For this review, take the finished solid that the model builds, in its own axes (mm). Face numbers are marked on the shaded views. A direction names the side the tool comes from. Round coordinates to 2 decimals unless told otherwise and drop trailing zeros. Loops run counter-clockwise (first coordinate to the right, second up) from the corner with the lowest first, then second, coordinate; pieces in that order, holes last. Notation, with made-up numbers: M -34,64 L 7,64 A11 ccw 7,70 Z; hole C -34,8.25 d11. An arc over 180 degrees is marked long. One line per question, with ' | ' between items. Start each with the question number.
1) We need section C-C (z = 24.5). Give the boundary of the cut face in (x, y).
2) We need section B-B (x = 10). Give the boundary of the cut face in (y, z), and give its area (3 significant figures).
3) For the marked faces 1, 2, 3 and 4, list the 3-axis set-ups (+Z, -Z, +X, -X, +Y, -Y) from which the entire face can be reached by the end or side of a thin tool; tool diameter is ignored.
4) For pin 1 Ø18.5 at (x, z) = (53.5, 31.5) entering from +Y; pin 2 Ø1.5 at (x, y) = (33.5, 7) entering from +Z; pin 3 Ø8.5 at (x, y) = (9.5, 6) entering from +Z, all flat-tipped, find the tip position at first contact; note any pin that passes through.
5) For probe 1 along Y at (x, z) = (10, 3); probe 2 along Z at (x, y) = (37, 75); probe 3 along Y at (x, z) = (17, 35), list the stretches that pass through material, from the lowest coordinate up. Write a range as from..to.
6) We need section D-D (z = 4). Give the boundary of the cut face in (x, y), and give its area (3 significant figures).
7) We need section A-A (y = 80). Give the boundary of the cut face in (x, z).
Autodesk Inventor part; units mm, degrees
ref_plane "YZ Plane" through (0, 0, 0) normal (1, 0, 0) x (0, 1, 0)
ref_plane "XZ Plane" through (0, 0, 0) normal (0, 1, 0) x (-1, 0, 0)
ref_plane "XY Plane" through (0, 0, 0) normal (0, 0, 1) x (1, 0, 0)
sketch "Sketch1" plane through (0, 0, 0) normal (0, 0, 1) x (1, 0, 0)
  line L0 (0, 0) -> (70, 0)
  line L1 (70, 0) -> (70, 90)
  line L2 (70, 90) -> (0, 90)
  line L3 (0, 90) -> (0, 0)
  dimension "d0" = 70
  dimension "d1" = 90
extrude "Extrusion1" add sketch "Sketch1" along normal blind 5
sketch "Sketch2" plane through (0, 0, 5) normal (0, 0, 1) x (1, 0, 0)
  circle A0 centre (35, 20) radius 12.5
  point P0 (0, 0)
  dimension "d4" = 25
extrude "Extrusion2" add sketch "Sketch2" along normal blind 40
sketch "Sketch3" plane through (35, 20, 45) normal (0, 0, 1) x (1, 0, 0)
  circle A0 centre (0, 0) radius 2.7
  point P0 (-35, -20)
  dimension "d7" = 5.4
extrude "Extrusion3" cut sketch "Sketch3" against normal blind 25
chamfer "Chamfer1" distance 4 angle 45 1 edges at (22.5, 20, 45) measured on face at (44.0861, 18.7875, 45)
sketch "Sketch4" plane through (0, 0, 5) normal (0, 0, 1) x (1, 0, 0)
  line L0 (0, 0) -> (70, 0)
  line L1 (32, 0) -> (38, 0)
  line L2 (38, 0) -> (38, 14)
  line L3 (38, 14) -> (32, 14)
  line L4 (32, 14) -> (32, 0)
  dimension "d13" = 6
  dimension "d14" = 14
extrude "Extrusion4" add sketch "Sketch4" along normal blind 36
chamfer "Chamfer2" distance 6 angle 45 1 edges at (35, 0, 41) measured on face at (35.3363, 2.5136, 41)
sketch "Sketch5" plane through (0, 0, 5) normal (0, 0, 1) x (1, 0, 0)
  line L0 (32, 72) -> (38, 72)
  line L1 (38, 72) -> (38, 27)
  line L2 (38, 27) -> (32, 27)
  line L3 (32, 27) -> (32, 72)
  line L4 (70, 0) -> (70, 90)
  line L5 (70, 23) -> (42, 23)
  line L6 (42, 23) -> (42, 17)
  line L7 (42, 17) -> (70, 17)
  line L8 (70, 17) -> (70, 23)
  line L9 (0, 90) -> (0, 0)
  line L10 (0, 23) -> (25.872, 23)
  line L11 (25.872, 23) -> (25.872, 17)
  line L12 (25.872, 17) -> (0, 17)
  line L13 (0, 17) -> (0, 23)
  dimension "d20" = 6
  dimension "d21" = 45
  dimension "d22" = 28
  dimension "d23" = 6
extrude "Extrusion5" add sketch "Sketch5" along normal blind 36
chamfer "Chamfer3" distance 20 angle 45 1 edges at (70, 20, 41) measured on face at (62.5, 20, 41)
chamfer "Chamfer4" distance 20 angle 45 1 edges at (0, 20, 41) measured on face at (7.5136, 20.3363, 41)
chamfer "Chamfer5" distance 35 angle 45 1 edges at (35, 72, 41) measured on face at (34, 72, 17)
sketch "Sketch6" plane through (0, 0, 5) normal (0, 0, 1) x (1, 0, 0)
  circle A0 centre (10, 7) radius 2.5
  circle A1 centre (60, 7) radius 2.5
  circle A2 centre (10, 80) radius 2.5
  circle A3 centre (60, 80) radius 2.5
  circle A4 centre (10, 45) radius 2.5
  circle A5 centre (60, 45) radius 2.5
  point P0 (0, 0)
  dimension "d35" = 5
  dimension "d36" = 5
  dimension "d37" = 5
  dimension "d38" = 5
  dimension "d39" = 5
  dimension "d40" = 5
extrude "Extrusion6" cut sketch "Sketch6" against normal blind 16
properties part number "wing_sail_base_1"
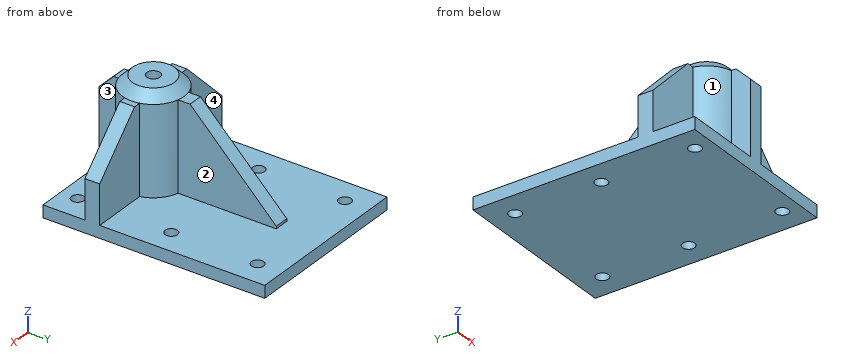
Answers below:
1) outline: M 3.5,17 L 22.87,17 A12.5 ccw 32,7.87 L 32,0 L 38,0 L 38,7.87 A12.5 ccw 47.13,17 L 66.5,17 L 66.5,23 L 47.13,23 A12.5 ccw 38,32.13 L 38,53.5 L 32,53.5 L 32,32.13 A12.5 ccw 22.87,23 L 3.5,23 Z; hole C 35,20 d5.4
2) outline: M 0,0 L 4.5,0 L 4.5,5 L 0,5 Z; M 9.5,0 L 42.5,0 L 42.5,5 L 23,5 L 23,31 L 17,31 L 17,5 L 9.5,5 Z; M 47.5,0 L 77.5,0 L 77.5,5 L 47.5,5 Z; M 82.5,0 L 90,0 L 90,5 L 82.5,5 Z | area: 531 mm^2
3) face 1: +Z, -X, -Y | face 2: +Z, +X, +Y | face 3: +Z, +X, -Y | face 4: +Z, -X, +Y
4) pin 1: y = 28.41 | pin 2: z = 41.16 | pin 3: z = 5
5) probe 1: 0..4.5, 9.5..42.5, 47.5..77.5, 82.5..90 | probe 2: 0..5 | probe 3: 17..23
6) outline: M 0,0 L 70,0 L 70,90 L 0,90 Z; hole C 10,7 d5; hole C 10,45 d5; hole C 10,80 d5; hole C 60,7 d5; hole C 60,45 d5; hole C 60,80 d5 | area: 6,180 mm^2
7) outline: M 0,0 L 7.5,0 L 7.5,5 L 0,5 Z; M 12.5,0 L 57.5,0 L 57.5,5 L 12.5,5 Z; M 62.5,0 L 70,0 L 70,5 L 62.5,5 Z
